Can you work these out from the drawing? Everything is in mm from the part's minimum corner. Give positions to 0.01 mm unless a question says otherwise; leave off trailing zeros. Write each loop counter-clockwise with the first axis right and the second up, starting at its lowest first coordinate (ties: lowest second). Pieces come first, ordered by that corner, then holes. Notation, with made-up numbers: (-26, 15.25) - (-10, 15.25) arc R33 cw to (-10, 44.25) - close; hole circle Ø10 at (-3, 67). An arc over 180 degrees is marked (long way). Write each question's results on one line, items separated by ' | '. Start each with the question number.
Item 1: Please list where these lines run through material, in increasing order: line 1 along Y through (x, z) = (5.7, 18.5); line 2 along X through (y, z) = (4.25, 11); line 3 along Y through (x, z) = (7, 9.25).
Item 2: Will these pins go through, and if not, where does the flat tip stop? P1, Ø4.5, axis at x = 5.7, y = 5.7, coming from the -Z side; P2, Ø6, axis at x = 1.5, z = 3.5, coming from the +Y side; P3, Ø1, axis at x = 9.5, z = 11, coming from the +Y side; P4, Ø3, axis at y = 7.5, z = 14.5, coming from the +X side.
Item 3: Suppose I cut it at A-A on y = 5.7. List the corners of the cut face in (x, z) for me, then the cut area to 3 significant figures.
Item 4: Suppose I cut it at C-C on z = 3.25. List the corners of the cut face in (x, y) for me.
Item 5: We'd pull the mould along X, two halves only. Please class the marked faces 1, 2 and 3: +X half, -X half, draft (parallel to the pull), parting line (faces both ways), or undercut.
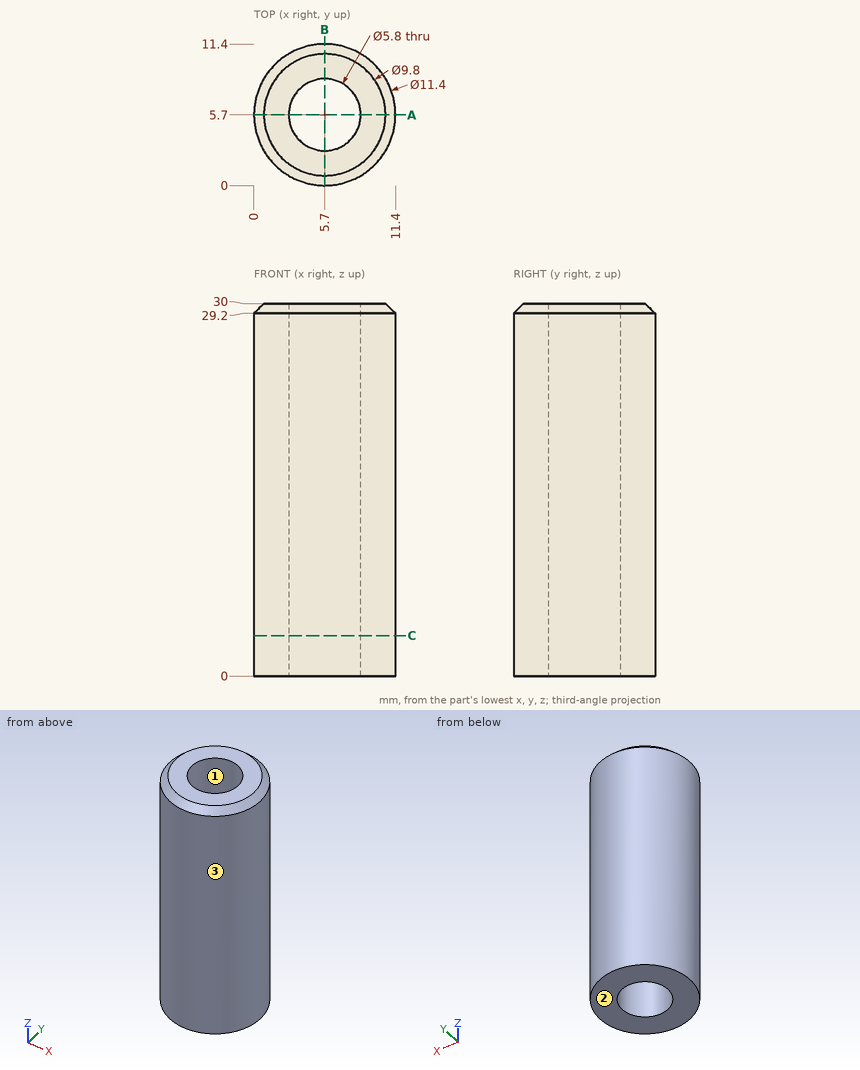
Checked values:
1) line 1: y = 0 to 2.8, 8.6 to 11.4 | line 2: x = 0.19 to 3.19, 8.21 to 11.21 | line 3: y = 0.15 to 3.11, 8.29 to 11.25
2) P1: passes through | P2: stops at y = 11.27 | P3: stops at y = 10.35 | P4: stops at x = 11.39
3) outline: (0, 0) - (2.8, 0) - (2.8, 30) - (0.8, 30) - (0, 29.2) - close; (8.6, 0) - (11.4, 0) - (11.4, 29.2) - (10.6, 30) - (8.6, 30) - close | area: 167 mm^2
4) outline: circle Ø11.4 at (5.7, 5.7); hole circle Ø5.8 at (5.7, 5.7)
5) face 1: undercut | face 2: draft | face 3: parting line
